from build123d import *

# Parameters (mm, degrees)
ESQUISSE1_W             = 27.85
ESQUISSE1_H             = 200
BOSS_EXTRU_2_DEPTH      = 6
ESQUISSE3_R             = 2.5
ENL_V_MAT_EXTRU_1_DEPTH = 6
ESQUISSE4_R             = 13.925
ENL_V_MAT_EXTRU_2_DEPTH = 3
ESQUISSE5_R             = 2.925
ENL_V_MAT_EXTRU_3_DEPTH = 3
ESQUISSE6_W             = 17.85
ESQUISSE6_H             = 23
ESQUISSE6_H_2           = 29
ENL_V_MAT_EXTRU_4_DEPTH = 10
CONG_1_R                = 10
CONG_2_R                = 10


with BuildPart() as part:
    # Esquisse1 → Boss.-Extru.2 (new body)
    with BuildSketch(Plane.XY):
        with Locations((1.835077519, -78.788662791)):
            Rectangle(ESQUISSE1_W, ESQUISSE1_H)
        with BuildLine():
            Line((-12.089922481, 21.211337209), (15.760077519, 21.211337209))
            ThreePointArc((15.760077519, 21.211337209), (1.835077519, 35.136337209), (-12.089922481, 21.211337209))
        make_face()
    extrude(amount=BOSS_EXTRU_2_DEPTH)

    # Esquisse3 → Enlèv. mat.-Extru.1 (cut)
    with BuildSketch(Plane.XY.offset(6)):
        with Locations((1.835077519, -170.788662791)):
            Circle(ESQUISSE3_R)
    extrude(amount=-ENL_V_MAT_EXTRU_1_DEPTH, mode=Mode.SUBTRACT)

    # Esquisse4 → Enlèv. mat.-Extru.2 (cut)
    with BuildSketch(Plane.XY.offset(6)):
        with Locations((1.835077519, 21.211337209)):
            Circle(ESQUISSE4_R)
    extrude(amount=-ENL_V_MAT_EXTRU_2_DEPTH, mode=Mode.SUBTRACT)

    # Esquisse5 → Enlèv. mat.-Extru.3 (cut)
    with BuildSketch(Plane.XY.offset(3)):
        with Locations((1.835077519, 21.211337209)):
            Circle(ESQUISSE5_R)
    extrude(amount=-ENL_V_MAT_EXTRU_3_DEPTH, mode=Mode.SUBTRACT)

    # Esquisse6 → Enlèv. mat.-Extru.4 (cut)
    with BuildSketch(Plane.XY.offset(6)):
        with BuildLine():
            Line((-7.089922481, -27.788662791), (10.760077519, -27.788662791))
            ThreePointArc((10.760077519, -27.788662791), (1.835077519, -18.863662791), (-7.089922481, -27.788662791))
        make_face()
        with Locations((1.835077519, -39.288662791)):
            Rectangle(ESQUISSE6_W, ESQUISSE6_H)
        with BuildLine():
            Line((-7.089922481, -50.788662791), (10.760077519, -50.788662791))
            ThreePointArc((10.760077519, -50.788662791), (1.835077519, -59.713662791), (-7.089922481, -50.788662791))
        make_face()
        with BuildLine():
            ThreePointArc((-7.089922481, -73.788662791), (1.835077519, -64.863662791), (10.760077519, -73.788662791))
            Line((10.760077519, -73.788662791), (-7.089922481, -73.788662791))
        make_face()
        with Locations((1.835077519, -88.288662791)):
            Rectangle(ESQUISSE6_W, ESQUISSE6_H_2)
        with BuildLine():
            Line((-7.089922481, -102.788662791), (10.760077519, -102.788662791))
            ThreePointArc((10.760077519, -102.788662791), (1.835077519, -111.713662791), (-7.089922481, -102.788662791))
        make_face()
        with BuildLine():
            Line((-7.089922481, -125.788662791), (10.760077519, -125.788662791))
            ThreePointArc((10.760077519, -125.788662791), (1.835077519, -116.863662791), (-7.089922481, -125.788662791))
        make_face()
        with Locations((1.835077519, -137.288662791)):
            Rectangle(ESQUISSE6_W, ESQUISSE6_H)
        with BuildLine():
            Line((-7.089922481, -148.788662791), (10.760077519, -148.788662791))
            ThreePointArc((10.760077519, -148.788662791), (1.835077519, -157.713662791), (-7.089922481, -148.788662791))
        make_face()
    extrude(amount=-ENL_V_MAT_EXTRU_4_DEPTH, mode=Mode.SUBTRACT)

    # Congé1
    cong_1_edges = [part.edges().sort_by_distance(p)[0] for p in [
        (-12.089922481, -178.788662791, 3),
    ]]
    fillet(cong_1_edges, radius=CONG_1_R)

    # Congé2
    cong_2_edges = [part.edges().sort_by_distance(p)[0] for p in [
        (15.760077519, -178.788662791, 3),
    ]]
    fillet(cong_2_edges, radius=CONG_2_R)


solid = part.part
Part model, mm, in its own coordinate system. A direction names the side the tool comes from. Coordinates: 2 decimals unless noted, no trailing zeros. Loops run counter-clockwise (first coordinate to the right, second up) from the corner with the lowest first, then second, coordinate; pieces in that order, holes last. Notation, with made-up numbers: M 62,8 L 70,8 A30 ccw 70,39 Z; hole C 48.5,34 d10. An arc over 180 degrees is marked long. Use a Markdown table: item, result. Add a question column.
Q1. Cut at B-B (x = 7.5). Write the cut outline in (y, z), and give its area (3 significant figures).
Q2. Probe L1, parallel to Y at x = 2, z = 2.2; L2, parallel to Y at x = -3.5, z = 4.9; L3, parallel to X at y = -73, z = 5.7 (3 decimals). List the from-to ranges inside material, lowest first.
Q3. Which spindle directions (+Z, -Z, +X, -X, +Y, -Y) get a long thin tool onto all of the face, cutting with end or side? Do faces 4 (the flat face through (10.76, -88, 3)), 5 (the cylindrical face through (12.75, -175.94, 3.04)), 6 (the flat face through (2, 25, 3)). Say none if no direction does.
Q4. Pin check, flat tips, straight feed: P1, Ø1, axis at x = 10.5, z = 2.5, coming from the +Y side; P2, Ø8.5, axis at x = 5.5, y = 20, coming from the +Z side. Stop position of each tip, or through.
Q5. Cut at D-D (y = -155.5). Write the cut outline in (x, z), and give its area (3 significant figures).
Q6. Cut at A-A (y = -34). Write the cut outline in (x, z), and give its area (3 significant figures).
Q7. Cut at C-C (z = 4.3). Write the cut outline in (x, y) (3 decimals), and give its area (3 significant figures).
Q8. Mould opens along Y. For faces 1 (the flat face through (2, -178.789, 3)), 2 (the flat face through (-8, -70, 0)), 3 (the cylindrical face through (2.03, -111.71, 3.04)) say: +Y half, -Y half, draft (parallel to the pull), parting line (faces both ways), or undercut.
Worked out:
| question | item | result |
|---|---|---|
| 1 | outline | M -178.64,0 L -155.69,0 L -155.69,6 L -178.64,6 Z; M -118.89,0 L -109.69,0 L -109.69,6 L -118.89,6 Z; M -66.89,0 L -57.69,0 L -57.69,6 L -66.89,6 Z; M -20.89,0 L 33.93,0 L 33.93,3 L 8.49,3 L 8.49,6 L -20.89,6 Z |
| 1 | area | 501 mm2 |
| 2 | L1 | y = -178.79 to -173.28, -168.29 to -157.71, -116.87 to -111.71, -64.87 to -59.71, -18.87 to 18.29, 24.13 to 35.14 |
| 2 | L2 | y = -178.69 to -155.94, -118.63 to -109.94, -66.63 to -57.94, -20.63 to 8.35 |
| 2 | L3 | x = -12.09 to -7.055, 10.725 to 15.76 |
| 3 | face 4 | +Z, -Z |
| 3 | face 5 | +Z, -Z, +X, -Y |
| 3 | face 6 | +Z, +Y |
| 4 | P1 | stops at y = 32.49 |
| 4 | P2 | stops at z = 3 |
| 5 | outline | M -12.09,0 L -4.05,0 L -4.05,6 L -12.09,6 Z; M 7.72,0 L 15.76,0 L 15.76,6 L 7.72,6 Z |
| 5 | area | 96.5 mm2 |
| 6 | outline | M -12.09,0 L -7.09,0 L -7.09,6 L -12.09,6 Z; M 10.76,0 L 15.76,0 L 15.76,6 L 10.76,6 Z |
| 6 | area | 60.0 mm2 |
| 7 | outline | M -12.09,-168.789 A10 ccw -2.09,-178.789 L 5.76,-178.789 A10 ccw 15.76,-168.789 L 15.76,21.211 A13.925 cw -12.09,21.211 Z; hole M -7.09,-148.789 A8.925 ccw 10.76,-148.789 L 10.76,-125.789 A8.925 ccw -7.09,-125.789 Z; hole M -7.09,-102.789 A8.925 ccw 10.76,-102.789 L 10.76,-73.789 A8.925 ccw -7.09,-73.789 Z; hole M -7.09,-50.789 A8.925 ccw 10.76,-50.789 L 10.76,-27.789 A8.925 ccw -7.09,-27.789 Z; hole C 1.835,-170.789 d5 |
| 7 | area | 3,110 mm2 |
| 8 | face 1 | -Y half |
| 8 | face 2 | draft |
| 8 | face 3 | undercut |
